Job drawing, mm, ordinate dimensions from the low corner. One solid piece. Round coordinates to 2 decimals unless told otherwise and drop trailing zeros. Order: outer loops, then holes, each group sorted by start corner. A loop starts at its lowest first (then second) coordinate and runs counter-clockwise, first axis right, second up. Notation, with made-up numbers: (45.25, -20) -> (69.25, -20) arc R21 cw to (69.25, -16) -> close; hole circle Ø10 at (16, 10). An arc over 180 degrees is marked (long way). Answer as a JSON object with one key per item and string values. Group by question number.
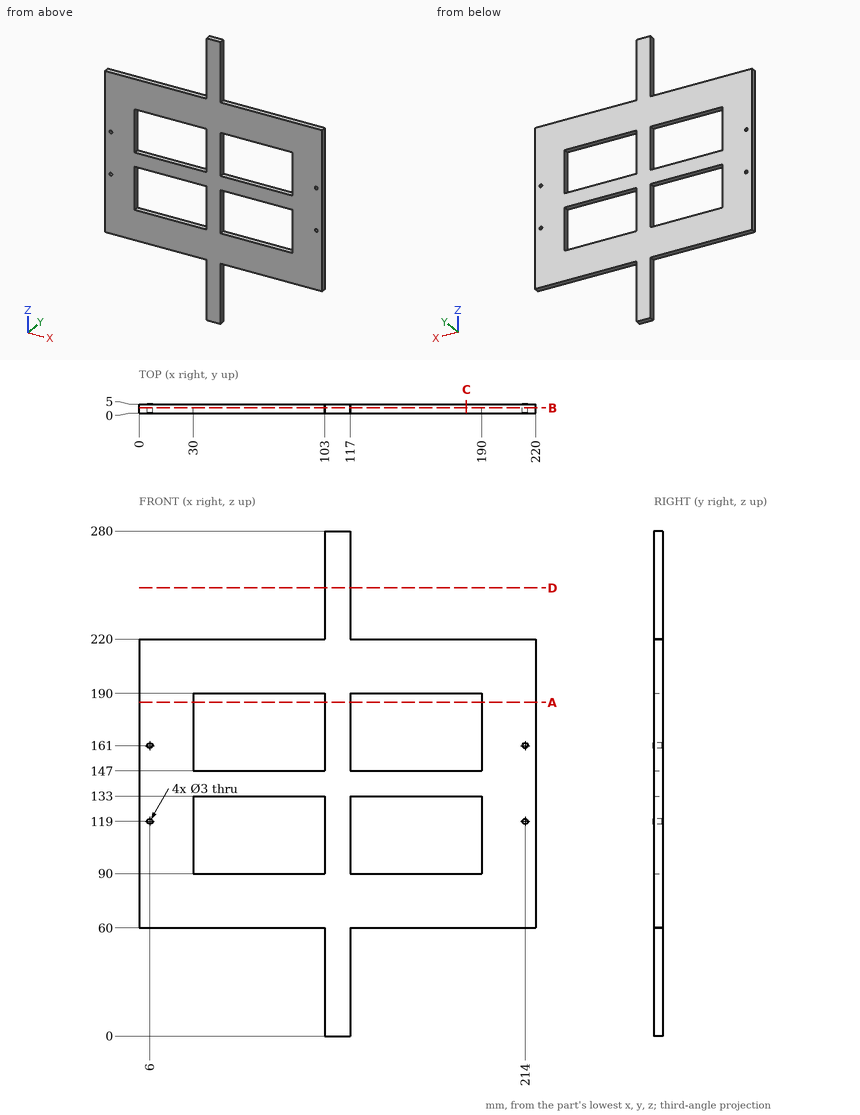
Q1. Band-saw the part on D-D (z = 248.5). List the corners of the cut face in (x, y), plus the area to 3 significant figures.
Q2. Band-saw the part on A-A (z = 185). List the corners of the cut face in (x, y), plus the area to 3 significant figures.
Q3. Drop flat-ended pins along their axis: pin 1 Ø3.5 at (x, z) = (6, 119) entering from +Y; pin 2 Ø1.5 at (y, z) = (1.5, 228.5) entering from +X; pin 3 Ø2.5 at (x, y) = (75.5, 3) entering from +Z; pin 4 Ø1.5 at (x, y) = (53.5, 3.5) entering from -Z. Give the stop position or say it passes through.
Q4. Wall check: line 1 (X direction, y = 2.9, z = 161); line 2 (Z direction, x = 140, y = 3.05); line 3 (X direction, y = 4.75, z = 183). Give the ranges that are in metal, low to high. Write a range as [from, to].
Q5. Band-saw the part on C-C (x = 181.5). List the corners of the cut face in (y, z).
Q6. Band-saw the part on B-B (y = 2.8). Count the separate pieces of the cut face and the enclosed holes in it, plus the area to 3 significant figures.
Completed:
{
 "1": {"outline": "(103, 0) -> (117, 0) -> (117, 5) -> (103, 5) -> close", "area": "70.0 mm2"},
 "2": {"outline": "(0, 0) -> (30, 0) -> (30, 5) -> (0, 5) -> close; (103, 0) -> (117, 0) -> (117, 5) -> (103, 5) -> close; (190, 0) -> (220, 0) -> (220, 5) -> (190, 5) -> close", "area": "370 mm2"},
 "3": {"pin 1": "y = 5", "pin 2": "x = 117", "pin 3": "z = 220", "pin 4": "z = 60"},
 "4": {"line 1": "[0, 4.5], [7.5, 30], [103, 117], [190, 212.5], [215.5, 220]", "line 2": "[60, 90], [133, 147], [190, 220]", "line 3": "[0, 30], [103, 117], [190, 220]"},
 "5": {"outline": "(0, 60) -> (5, 60) -> (5, 90) -> (0, 90) -> close; (0, 133) -> (5, 133) -> (5, 147) -> (0, 147) -> close; (0, 190) -> (5, 190) -> (5, 220) -> (0, 220) -> close"},
 "6": {"separate pieces": "1", "enclosed holes": "8", "area": "24,300 mm2"}
}
